```python
from build123d import *

# Parameters (mm, degrees)
F1_DEPTH = 6.35
F0_W     = 116.84
F0_H     = 6.35
F2_DEPTH = 25.4
F3_R     = 5.08
F4_W     = 48.26
F4_H     = 8.89
F5_DEPTH = 25.4
F6_R     = 5.08
F7_R     = 1.35255
F8_DEPTH = 12.7


with BuildPart() as f1:
    # F0 (on Front) → F1 (new body, symmetric)
    with BuildSketch(Plane.XZ):
        with BuildLine():
            ThreePointArc((4.7625, 0), (0, -4.7625), (-4.7625, 0))
            Line((-4.7625, 0), (-8.89, 0))
            Line((-8.89, 0), (-8.89, -39.37))
            Line((-8.89, -39.37), (107.95, -39.37))
            Line((107.95, -39.37), (107.95, 0))
            Line((107.95, 0), (102.235, 0))
            ThreePointArc((102.235, 0), (99.06, -3.175), (95.885, 0))
            Line((95.885, 0), (90.17, 0))
            Line((90.17, 0), (90.17, -26.67))
            ThreePointArc((90.17, -26.67), (88.310128, -31.160128), (83.82, -33.02))
            Line((83.82, -33.02), (81.28, -33.02))
            ThreePointArc((81.28, -33.02), (76.789872, -31.160128), (74.93, -26.67))
            Line((74.93, -26.67), (74.93, 0))
            Line((74.93, 0), (69.215, 0))
            ThreePointArc((69.215, 0), (66.04, -3.175), (62.865, 0))
            Line((62.865, 0), (57.15, 0))
            Line((57.15, 0), (57.15, -26.67))
            ThreePointArc((57.15, -26.67), (55.290128, -31.160128), (50.8, -33.02))
            Line((50.8, -33.02), (48.26, -33.02))
            ThreePointArc((48.26, -33.02), (43.769872, -31.160128), (41.91, -26.67))
            Line((41.91, -26.67), (41.91, 0))
            Line((41.91, 0), (37.7825, 0))
            ThreePointArc((37.7825, 0), (33.02, -4.7625), (28.2575, 0))
            Line((28.2575, 0), (24.13, 0))
            Line((24.13, 0), (24.13, -26.67))
            ThreePointArc((24.13, -26.67), (22.270128, -31.160128), (17.78, -33.02))
            Line((17.78, -33.02), (15.24, -33.02))
            ThreePointArc((15.24, -33.02), (10.749872, -31.160128), (8.89, -26.67))
            Line((8.89, -26.67), (8.89, 0))
            Line((8.89, 0), (4.7625, 0))
        make_face()
    extrude(amount=F1_DEPTH, both=True)

    # F0 (on Front) → F2 (join, symmetric)
    with BuildSketch(Plane.XZ):
        with Locations((49.53, -42.545)):
            Rectangle(F0_W, F0_H)
    extrude(amount=F2_DEPTH, both=True)

    # F3
    f3_edges = [f1.edges().sort_by_distance(p)[0] for p in [
        (49.53, -6.35, -39.37),
        (49.53, 6.35, -39.37),
        (107.95, -25.4, -42.545),
        (-8.89, -25.4, -42.545),
        (107.95, 25.4, -42.545),
        (-8.89, 25.4, -42.545),
    ]]
    fillet(f3_edges, radius=F3_R)

    # F4 (on face) → F5 (cut)
    with BuildSketch(Plane(origin=(0, 0, -45.72), x_dir=(1, 0, 0), z_dir=(0, 0, -1))):
        with Locations((20.32, 15.875)):
            Rectangle(F4_W, F4_H)
        with Locations((78.74, 15.875)):
            Rectangle(F4_W, F4_H)
        with Locations((78.74, -15.875)):
            Rectangle(F4_W, F4_H)
        with Locations((20.32, -15.875)):
            Rectangle(F4_W, F4_H)
    extrude(amount=-F5_DEPTH, mode=Mode.SUBTRACT)

    # F6
    f6_edges = [f1.edges().sort_by_distance(p)[0] for p in [
        (-3.81, 20.32, -42.545),
        (102.87, 20.32, -42.545),
        (-3.81, -20.32, -42.545),
        (102.87, -20.32, -42.545),
    ]]
    fillet(f6_edges, radius=F6_R)

    # F7 (on face) → F8 (cut)
    with BuildSketch(Plane.XY):
        with Locations((60.0075, 0)):
            Circle(F7_R)
    extrude(amount=-F8_DEPTH, mode=Mode.SUBTRACT)


solid = f1.part
```
For this review, take the finished solid that the model builds, in its own axes (mm). A direction names the side the tool comes from. Round coordinates to 2 decimals unless told otherwise and drop trailing zeros. Write each loop counter-clockwise with the first axis right and the second up, starting at its lowest first coordinate (ties: lowest second). Pieces come first, ordered by that corner, then holes. Notation, with made-up numbers: (74, -11) - (115, -11) arc R16 ccw to (115, 12) - close; hole circle Ø4 at (-1, 89). An arc over 180 degrees is marked (long way). Answer as CSV lines item,"result". Start each with the question number.
(1) Mouldability with a two-part tool opening along Y and no side actions: class faces 4 (the cylindrical face through (-2.282, 18.871, -42.501)), 5 (the flat face through (8.89, 0, -14)), 6 (the cylindrical face through (50.348, -7.878, -37.921)) as +Y half, -Y half, draft (parallel to the pull), parting line (faces both ways), or undercut.
(2) For pin 1 (4 mm diameter, centred on x = 75.5, y = -18, fed in from +Z); pin 2 (2 mm diameter, centred on x = 72.5, z = -33, fed in from -Y), all flat-tipped, find the tip position at first contact; note any pin that passes through.
(3) Add section B-B, the plane x = 66.04. State the section outline as (y, z) points (3 decimals), plus the area to 3 significant figures.
(4) Add section A-A, the plane z = -8.5. State the section outline as (x, y) points.
(5) Machinability: for faces 1 (the cylindrical face through (101.342, 18.871, -42.501)), 2 (the flat face through (62, -6.35, -21)), 3 (the flat face through (74.93, 0, -14)), which of the approach directions +Z, -Z, +X, -X, +Y, -Y give a long, thin tool a straight path to every point of the face, cutting with its end or side? Answer none if there is none.
(6) Add section D-D, the plane z = -15.5. State the section outline as (x, y) points.
(7) Add section C-C, the plane y = -13.5. State the section outline as (x, z) points.
(8) For line 1 (X direction, y = -2, z = -5); line 2 (Y direction, x = 64, z = -40); line 3 (X direction, y = 16, z = -42), list the stretches that pass through material, from the lowest coordinate up.
From the geometry:
1,face 4,"undercut"
1,face 5,"draft"
1,face 6,"-Y half"
2,pin 1,"passes through"
2,pin 2,"stops at y = -6.35"
3,outline,"(-25.4, -45.72) - (-20.32, -45.72) - (-20.32, -39.37) - (-25.4, -39.37) - close; (-11.43, -45.72) - (11.43, -45.72) - (11.43, -39.37) arc R5.08 cw to (6.35, -34.29) - (6.35, -3.175) - (-6.35, -3.175) - (-6.35, -34.29) arc R5.08 cw to (-11.43, -39.37) - close; (20.32, -45.72) - (25.4, -45.72) - (25.4, -39.37) - (20.32, -39.37) - close"
3,area,"680 mm²"
4,outline,"(-8.89, -6.35) - (8.89, -6.35) - (8.89, 6.35) - (-8.89, 6.35) - close; (24.13, -6.35) - (41.91, -6.35) - (41.91, 6.35) - (24.13, 6.35) - close; (57.15, -6.35) - (74.93, -6.35) - (74.93, 6.35) - (57.15, 6.35) - close; (90.17, -6.35) - (107.95, -6.35) - (107.95, 6.35) - (90.17, 6.35) - close; hole circle Ø2.71 at (60.01, 0)"
5,face 1,"+Z, -Z"
5,face 2,"+Z, +X, -X, -Y"
5,face 3,"+Z, +Y, -Y"
6,outline,"(-8.89, -6.35) - (8.89, -6.35) - (8.89, 6.35) - (-8.89, 6.35) - close; (24.13, -6.35) - (41.91, -6.35) - (41.91, 6.35) - (24.13, 6.35) - close; (57.15, -6.35) - (74.93, -6.35) - (74.93, 6.35) - (57.15, 6.35) - close; (90.17, -6.35) - (107.95, -6.35) - (107.95, 6.35) - (90.17, 6.35) - close"
7,outline,"(-8.89, -45.72) - (-3.81, -45.72) - (-3.81, -39.37) - (-8.89, -39.37) - close; (44.45, -45.72) - (54.61, -45.72) - (54.61, -39.37) - (44.45, -39.37) - close; (102.87, -45.72) - (107.95, -45.72) - (107.95, -39.37) - (102.87, -39.37) - close"
8,line 1,"x = -8.89 to 8.89, 24.13 to 41.91, 57.15 to 74.93, 90.17 to 107.95"
8,line 2,"y = -25.4 to -20.32, -11.43 to 11.43, 20.32 to 25.4"
8,line 3,"x = -8.89 to -3.75, 44.45 to 54.61, 102.81 to 107.95"
